Can you work these out from the model? Positions are in its coordinate system, mm. Face numbers are marked on the shaded views. A direction names the side the tool comes from. Coordinates: 2 decimals unless noted, no trailing zeros. Order: outer loops, then holes, each group sorted by start corner. A loop starts at its lowest first (then second) coordinate and runs counter-clockwise, first axis right, second up. Notation, with made-up numbers: (-6.75, -37.5) - (31.25, -37.5) arc R25 cw to (31.25, -0.5) - close; hole circle Ø9 at (36, 80.25). An arc over 180 degrees is marked (long way). Use a Markdown table: item, result. Add a question column.
(1) On a 3-axis mill with a long thin cutter (end or side, diameter ignored), from which of +Z, -Z, +X, -X, +Y, -Y can I reach the whole of each face in a straight line? I mean the marked faces 1, 2 and 3. Say none if no direction works.
(2) If I drill on L1, parallel to Y at x = 10.5, z = 13; L2, parallel to Y at x = -4, z = 24.5; L3, parallel to Y at x = -46, z = 25.5, over which ranges is the centre line in solid material (lowest first)? Write a range as [from, to].
(3) I want a section at B-B (x = -31.5). List the corners of the cut face in (y, z) for me.
(4) For pin 1 Ø6 at (x, y) = (17.5, 4) entering from -Z; pin 2 Ø1 at (x, z) = (-3, 9) entering from +Y; pin 3 Ø1 at (y, z) = (14.5, 39.5) entering from -X, each with a flat end and sliding along its axis, tell me the tip position at first contact or that it passes through.
(5) I want a section at A-A (x = 9.5). List the corners of the cut face in (y, z) for me.
(6) We'd pull the mould along X, two halves only. Please class the marked faces 4, 5 and 6: pulls with the +X half, pulls with the -X half, needs draft (parallel to the pull), parting line crosses it, or undercut.
(7) I want a section at C-C (x = -20.5). List the corners of the cut face in (y, z) for me, and give its area (3 significant figures).
```python
from build123d import *

# Parameters (mm, degrees)
F1_DEPTH    = 50
F2_T1_DEPTH = 61.9175359259
F2_T3_DEPTH = 58.3909963118
F2_T5_DEPTH = 60
F3_W        = 4.27056849
F3_H        = 50
F4_DEPTH    = 1
F5_SIZE     = 0.99999


# Not quite as in the source:
# - a fillet or chamfer that OpenCascade refuses, or shapes differently, is made with other operations: its cross-section is extruded or revolved along the edge and cut away or added
# - a fillet or chamfer is up to 0.001 mm smaller than in the source, because OpenCascade refuses the exact size


with BuildPart() as f1:
    # F0 (on Top) → F1 (new body)
    with BuildSketch(Plane.XY):
        Polygon((-53.1016754424, 0), (46.8983245576, 0), (46.8983245576, 3), (-19.0739845247, 3), (46.8983245576, 14.6326980708), (46.8983245576, 17.6326980708), align=None)
    extrude(amount=F1_DEPTH)

    # F2: fillet of radius 2 on 4 edges, made by hand

    # F2_s2 → F2_t1 (cut)
    with BuildSketch(Plane.XY.offset(-5.958767963)):
        with BuildLine():
            ThreePointArc((44.5510282023, 17.2188063917), (46.183899777, 16.7812797719), (46.8983245576, 15.2491908857))
            Line((46.8983245576, 15.2491908857), (46.8983245576, 17.6326980708))
            Line((46.8983245576, 17.6326980708), (44.5510282023, 17.2188063917))
        make_face()
    extrude(amount=F2_T1_DEPTH, mode=Mode.SUBTRACT)

    # F2_s4 → F2_t3 (cut)
    with BuildSketch(Plane.XY.offset(-4.1954981559)):
        with BuildLine():
            ThreePointArc((45.245620913, 14.3412818272), (46.4304134439, 15.0253221138), (46.8983245576, 16.3108973332))
            Line((46.8983245576, 16.3108973332), (46.8983245576, 14.6326980708))
            Line((46.8983245576, 14.6326980708), (45.245620913, 14.3412818272))
        make_face()
    extrude(amount=F2_T3_DEPTH, mode=Mode.SUBTRACT)

    # F2_s6 → F2_t5 (cut)
    with BuildSketch(Plane.XY.offset(-5)):
        with BuildLine():
            ThreePointArc((46.8983245576, 1), (46.31253812, 2.4142135624), (44.8983245576, 3))
            Line((44.8983245576, 3), (46.8983245576, 3))
            Line((46.8983245576, 3), (46.8983245576, 1))
        make_face()
        with BuildLine():
            ThreePointArc((44.8983245576, 0), (46.31253812, 0.5857864376), (46.8983245576, 2))
            Line((46.8983245576, 2), (46.8983245576, 0))
            Line((46.8983245576, 0), (44.8983245576, 0))
        make_face()
    extrude(amount=F2_T5_DEPTH, mode=Mode.SUBTRACT)

    # F3 (on face) → F4 (join)
    with BuildSketch(Plane(origin=(-1.6012114389, 9.0809213228, 0), x_dir=(-0.984807753, -0.1736481777, 0), z_dir=(-0.1736481777, 0.984807753, 0))):
        with Locations((45.5371029675, 25)):
            Rectangle(F3_W, F3_H)
        with Locations((35.1371029675, 25)):
            Rectangle(F3_W, F3_H)
        with Locations((24.7371029675, 25)):
            Rectangle(F3_W, F3_H)
        with Locations((14.3371029675, 25)):
            Rectangle(F3_W, F3_H)
        with Locations((3.9371029675, 25)):
            Rectangle(F3_W, F3_H)
        with Locations((-6.4628970325, 25)):
            Rectangle(F3_W, F3_H)
        with Locations((-16.8628970325, 25)):
            Rectangle(F3_W, F3_H)
        with Locations((-27.2628970325, 25)):
            Rectangle(F3_W, F3_H)
        with Locations((-37.6628970325, 25)):
            Rectangle(F3_W, F3_H)
    extrude(amount=F4_DEPTH)

    # F5 (size 1 in the source; OpenCascade refuses exactly that, so slightly less here)
    f5_edges = [f1.edges().sort_by_distance(p)[0] for p in [
        (-48.722996, 1.787506, 25),
        (-44.517307, 2.529082, 25),
        (-38.480996, 3.593447, 25),
        (-34.275307, 4.335023, 25),
        (-28.238995, 5.399388, 25),
        (-24.033306, 6.140964, 25),
        (-17.996994, 7.205329, 25),
        (-13.791305, 7.946905, 25),
        (-7.754994, 9.01127, 25),
        (-3.549305, 9.752847, 25),
        (2.487007, 10.817211, 25),
        (6.692696, 11.558788, 25),
        (12.729008, 12.623152, 25),
        (16.934697, 13.364729, 25),
        (22.971008, 14.429093, 25),
        (27.176697, 15.17067, 25),
        (33.213009, 16.235034, 25),
        (37.418698, 16.976611, 25),
    ]]
    chamfer(f5_edges, length=F5_SIZE)


solid = f1.part
```
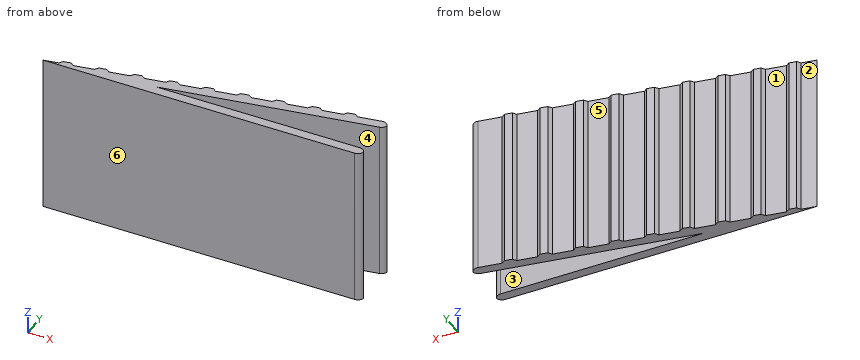
Answers follow:
| question | item | result |
|---|---|---|
| 1 | face 1 | +Z, -Z, +Y |
| 1 | face 2 | +Z, -Z, -X, +Y |
| 1 | face 3 | +Z, -Z, +X |
| 2 | L1 | y = [0, 3], [8.21, 11.21] |
| 2 | L2 | y = [0, 3], [5.66, 9.21] |
| 2 | L3 | y = [0, 2.27] |
| 3 | outline | (0, 0) - (3.81, 0) - (3.81, 50) - (0, 50) - close |
| 4 | pin 1 | stops at z = 0 |
| 4 | pin 2 | stops at y = 8.92 |
| 4 | pin 3 | stops at x = 23.53 |
| 5 | outline | (0, 0) - (3, 0) - (3, 50) - (0, 50) - close; (8.04, 0) - (11.04, 0) - (11.04, 50) - (8.04, 50) - close |
| 6 | face 4 | pulls with the +X half |
| 6 | face 5 | undercut |
| 6 | face 6 | needs draft |
| 7 | outline | (0, 0) - (5.75, 0) - (5.75, 50) - (0, 50) - close |
| 7 | area | 287 mm² |
